The figure shows three views and two pictorial views of one solid part (mm, origin at its lowest corner). Answer the questions. A direction names the side the tool comes from. Coordinates: 2 decimals unless noted, no trailing zeros. Loops run counter-clockwise (first coordinate to the right, second up) from the corner with the lowest first, then second, coordinate; pieces in that order, holes last. Notation, with made-up numbers: (56.25, 39.25) -> (68.25, 39.25) arc R21 ccw to (68.25, 52.25) -> close; hole circle Ø5 at (61.25, 68.25). An arc over 180 degrees is marked (long way). Answer in a Markdown table with one row per item.
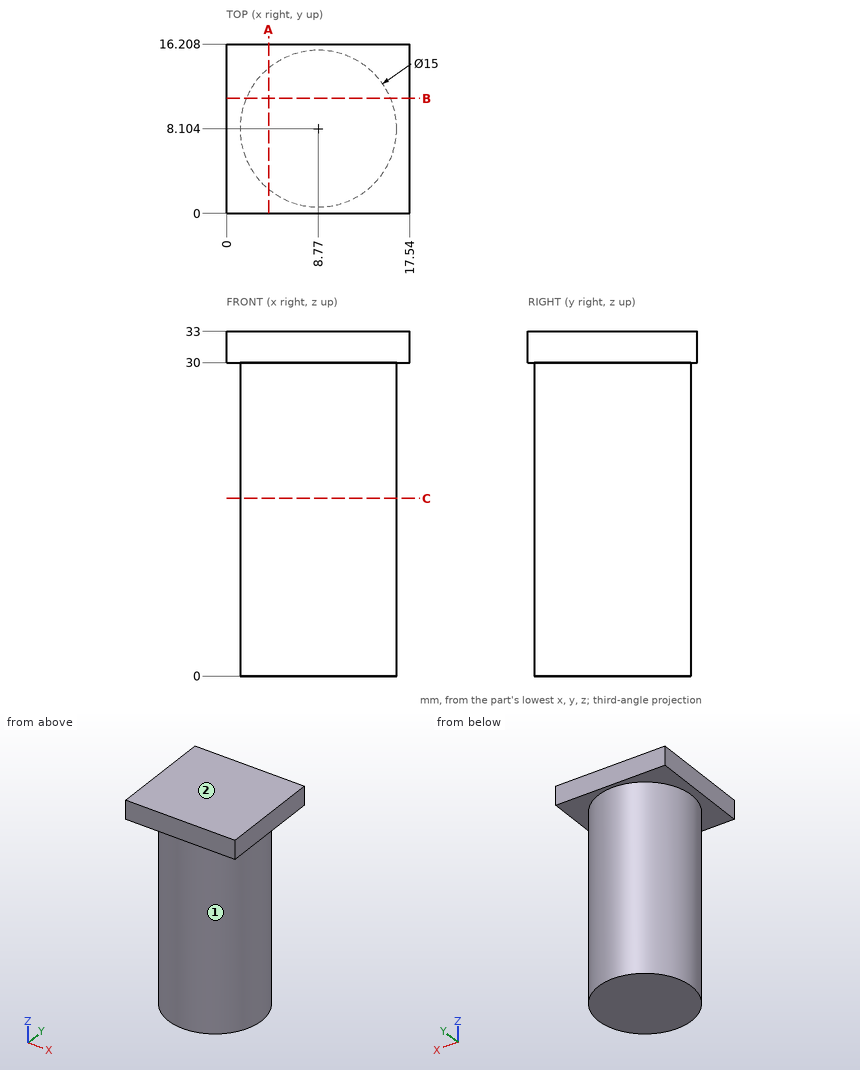
Item 1: Find the intervals of material crossed by probe 1 along X at (y, z) = (8.25, 16); probe 2 along Z at (x, y) = (1, 11.5); probe 3 along Y at (x, z) = (8.5, 26), in increasing order.
Findings below:
| item | result |
|---|---|
| probe 1 | x = 1.27 to 16.27 |
| probe 2 | z = 30 to 33 |
| probe 3 | y = 0.61 to 15.6 |
Item 2: A cutting plane is placed at C-C, the plane z = 17. Determine the outline of the cut face in (x, y) (1 decimal).
Findings below:
| item | result |
|---|---|
| outline | circle Ø15 at (8.8, 8.1) |
Item 3: A tool of negligible diameter and unlimited length cuts with its end or side. For the marked faces 1 and 2, from which of +Z, -Z, +X, -X, +Y, -Y can it reach the whole face along a straight path? Write none if from no direction.
Findings below:
| item | result |
|---|---|
| face 1 | -Z |
| face 2 | +Z, +X, -X, +Y, -Y |
Item 4: Flat-ended cylindrical pins translate along their axes: pin 1 Ø4 at (x, y) = (14, 5.5) entering from -Z; pin 2 Ø3 at (y, z) = (3, 19.5) entering from +X; pin 3 Ø1 at (y, z) = (13, 16) entering from +X; pin 4 Ø4 at (y, z) = (3.5, 12.5) entering from +X. Find the tip coordinate at first contact, or state that the pin passes through.
Findings below:
| item | result |
|---|---|
| pin 1 | stops at z = 0 |
| pin 2 | stops at x = 15.35 |
| pin 3 | stops at x = 14.85 |
| pin 4 | stops at x = 15.8 |
Item 5: A cutting plane is placed at B-B, the plane y = 11. Determine the outline of the cut face in (x, z), plus the area to 3 significant figures.
Findings below:
| item | result |
|---|---|
| outline | (0, 30) -> (1.85, 30) -> (1.85, 0) -> (15.69, 0) -> (15.69, 30) -> (17.54, 30) -> (17.54, 33) -> (0, 33) -> close |
| area | 468 mm2 |
Item 6: A cutting plane is placed at A-A, the plane x = 4. Determine the outline of the cut face in (y, z), plus the area to 3 significant figures.
Findings below:
| item | result |
|---|---|
| outline | (0, 30) -> (2.32, 30) -> (2.32, 0) -> (13.89, 0) -> (13.89, 30) -> (16.21, 30) -> (16.21, 33) -> (0, 33) -> close |
| area | 396 mm2 |
